from build123d import *

# Parameters (mm, degrees)
F0_R     = 9
F1_DEPTH = 60
F2_R     = 15
F2_R_2   = 9
F3_DEPTH = 5
F4_R     = 3.5
F5_DEPTH = 10


with BuildPart() as f1:
    # F0 (on Front) → F1 (new body)
    with BuildSketch(Plane.XZ):
        Circle(F0_R)
    extrude(amount=F1_DEPTH)

    # F2 (on face) → F3 (join)
    with BuildSketch(Plane.XZ.offset(60)):
        Circle(F2_R)
        Circle(F2_R_2, mode=Mode.SUBTRACT)
        Circle(F2_R_2)
    extrude(amount=F3_DEPTH)

    # F4 (on face) → F5 (cut)
    with BuildSketch(Plane.XZ.offset(65)):
        with Locations((0, 10)):
            Circle(F4_R)
    extrude(amount=-F5_DEPTH, mode=Mode.SUBTRACT)


solid = f1.part
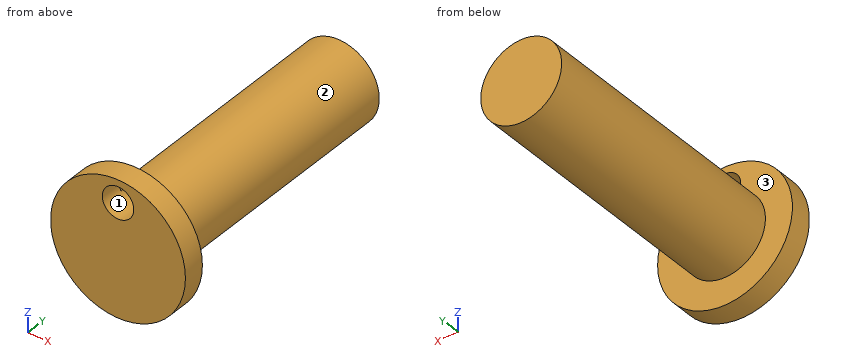
Source: CAD feature listing. Evaluate the final solid. Frame: model axes, mm. Face numbers are marked on the shaded views. Coordinates: 2 decimals unless noted, no trailing zeros. Loops run counter-clockwise (first coordinate to the right, second up) from the corner with the lowest first, then second, coordinate; pieces in that order, holes last. Notation, with made-up numbers: (33, 60.5) - (80, 60.5) arc R29 ccw to (80, 86.5) - close; hole circle Ø8 at (-15, 57.5). An arc over 180 degrees is marked (long way). One line per question, with ' | ' between items.
1) Pull-direction query (X, two-part tool) for the marked faces 1, 2 and 3; classes: released by +X, released by -X, zero draft, split by the parting line, or undercut.
Report:
face 1: undercut | face 2: split by the parting line | face 3: zero draft
2) Section D-D, the plane y = -38. Return loops of the section in (x, z), then the cut area to 3 significant figures.
Report:
outline: circle Ø18 at (0, 0) | area: 254 mm²
3) First-contact query: P1, Ø10, axis at x = -5.5, y = -30.5, coming from the -Z side; P2, Ø4, axis at x = 8.5, z = 11, coming from the +Y side; P3, Ø6, axis at y = -44.5, z = 6, coming from the +X side; P4, Ø1.5, axis at y = -50, z = 10, coming from the -X side. Flat tips, straight axial feed; report the tip coordinate or a pass-through.
Report:
P1: stops at z = -8.99 | P2: stops at y = -60 | P3: stops at x = 8.49 | P4: passes through
4) Section C-C, the plane z = 0. Return loops of the section in (x, y), then the cut area to 3 significant figures.
Report:
outline: (-15, -65) - (15, -65) - (15, -60) - (9, -60) - (9, 0) - (-9, 0) - (-9, -60) - (-15, -60) - close | area: 1,230 mm²
5) Section A-A, the plane x = 0. Return loops of the section in (y, z).
Report:
outline: (-65, -15) - (-60, -15) - (-60, -9) - (0, -9) - (0, 9) - (-55, 9) - (-55, 6.5) - (-65, 6.5) - close; (-65, 13.5) - (-60, 13.5) - (-60, 15) - (-65, 15) - close
6) Line query: line 1 along Z through (x, y) = (0, -60.5); line 2 along Y through (x, z) = (4.25, -11.75); line 3 along Z through (x, y) = (0, -59). Output: solid intervals per line, ascending.
Report:
line 1: z = -15 to 6.5, 13.5 to 15 | line 2: y = -65 to -60 | line 3: z = -9 to 6.5
7) Section B-B, the plane z = 10. Return loops of the section in (x, y).
Report:
outline: (-11.18, -65) - (-3.5, -65) - (-3.5, -60) - (-11.18, -60) - close; (3.5, -65) - (11.18, -65) - (11.18, -60) - (3.5, -60) - close
